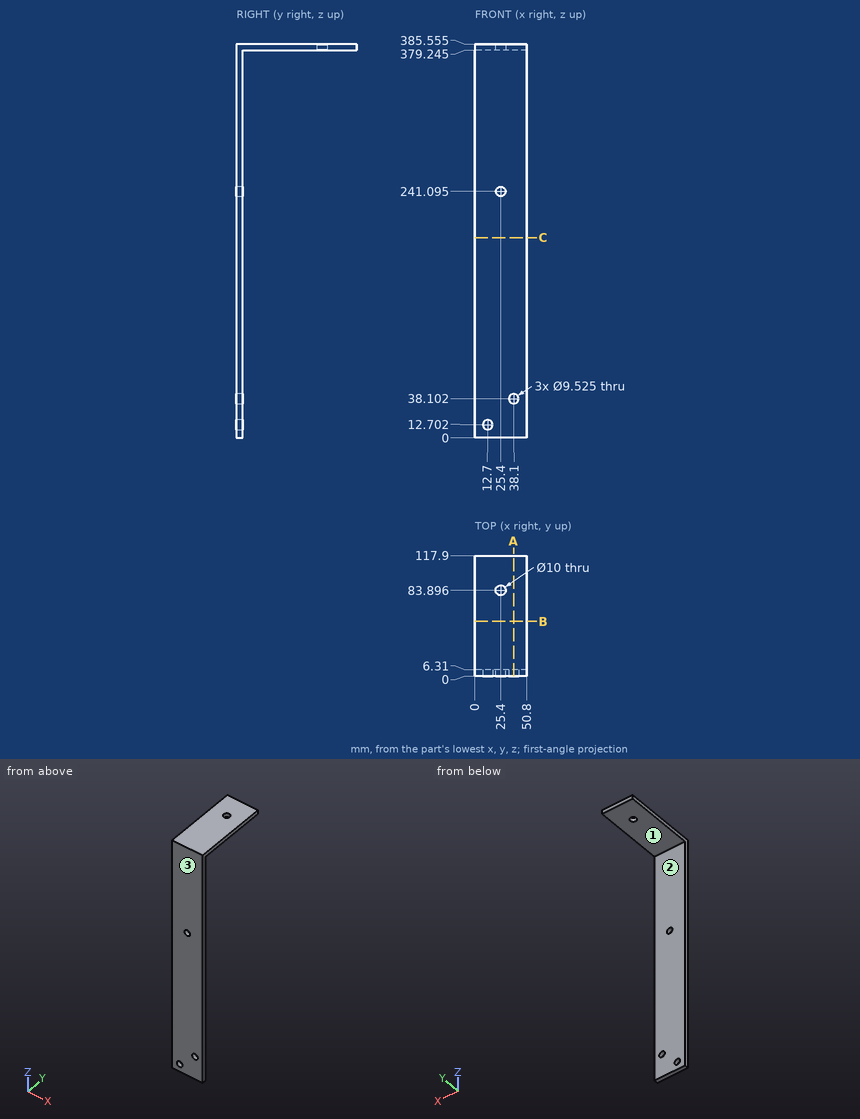
For this review, use the dimensioned drawing (mm, ordinates from the lowest corner) and the shaded views. Round coordinates to 2 decimals unless told otherwise and drop trailing zeros. Loops run counter-clockwise (first coordinate to the right, second up) from the corner with the lowest first, then second, coordinate; pieces in that order, holes last. Notation, with made-up numbers: M 83,65.25 L 101,65.25 A11 ccw 101,76.25 Z; hole C 58.25,60.5 d5. An arc over 180 degrees is marked long. Answer as a JSON object with one key per item and string values.
(1) Take a section at C-C on z = 196. Give the boundary of the cut face in (x, y).
Resolved:
{"outline": "M 0,0 L 50.8,0 L 50.8,6.31 L 0,6.31 Z"}
(2) To check wall thickness, follow line 1 along Y through (x, z) = (25.4, 382); line 2 along Y through (x, z) = (26.5, 123.5); line 3 along Z through (x, y) = (12, 42) (1 decimal). State the ranges of each line that lie inside material, in increasing order.
Resolved:
{"line 1": "0 to 78.9, 88.9 to 117.9", "line 2": "0 to 6.31", "line 3": "379.2 to 385.6"}
(3) Take a section at B-B on y = 53.5. Give the boundary of the cut face in (x, z) (1 decimal).
Resolved:
{"outline": "M 0,379.2 L 50.8,379.2 L 50.8,385.6 L 0,385.6 Z"}
(4) Take a section at A-A on x = 38.1. Give the boundary of the cut face in (y, z) (1 decimal).
Resolved:
{"outline": "M 0,0 L 6.3,0 L 6.3,33.3 L 0,33.3 Z; M 0,42.9 L 6.3,42.9 L 6.3,379.2 L 117.9,379.2 L 117.9,385.6 L 0,385.6 Z"}
(5) Clearance check with flat-ended pins moving along their axes: P1, Ø12, axis at x = 9, z = 282.5, coming from the +Y side; P2, Ø15, axis at x = 13.5, y = 56, coming from the -Z side (3 decimals). State where each tip first meets the part, or that it passes through.
Resolved:
{"P1": "y = 6.31", "P2": "z = 379.245"}
(6) Draft analysis for pull direction Y (two halves, no side actions). For the marked faces 1, 2 and 3, state which applies: released by +Y, released by -Y, zero draft, split by the parting line, or undercut.
Resolved:
{"face 1": "zero draft", "face 2": "released by +Y", "face 3": "released by -Y"}
